Read the model definition and answer for the solid it produces. Units are mm, in the model's axes. Face numbers are marked on the shaded views. Coordinates: 2 decimals unless noted, no trailing zeros. Order: outer loops, then holes, each group sorted by start corner. A loop starts at its lowest first (then second) coordinate and runs counter-clockwise, first axis right, second up. Notation, with made-up numbers: (-13, 63.5) - (32, 63.5) arc R21 ccw to (32, 93.5) - close; hole circle Ø11 at (66, -16). An arc over 180 degrees is marked (long way). Write item = value, one per line.
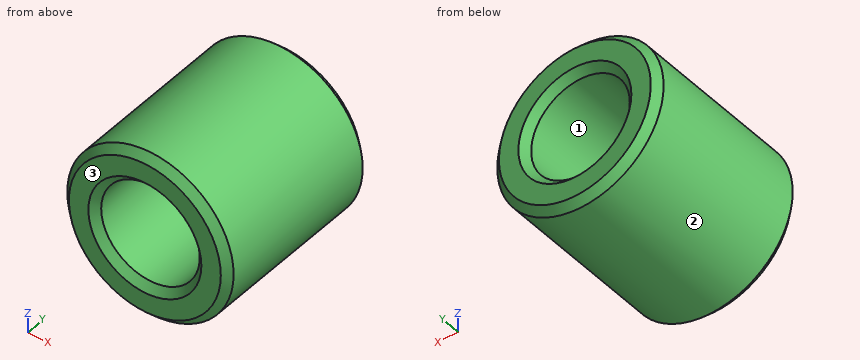
from build123d import *

# Parameters (mm, degrees)
F0_R     = 58.497005
F1_DEPTH = 127
F2_R     = 34.670049
F3_DEPTH = 127.001
F4_SIZE  = 5.08


with BuildPart() as f1:
    # F0 (on Front) → F1 (new body)
    with BuildSketch(Plane.XZ):
        Circle(F0_R)
    extrude(amount=F1_DEPTH)

    # F2 (on face) → F3 (cut, through all)
    with BuildSketch(Plane(origin=(0, 0, 0), x_dir=(-1, 0, 0), z_dir=(0, 1, 0))):
        Circle(F2_R)
    extrude(amount=-F3_DEPTH, mode=Mode.SUBTRACT)

    # F4
    f4_edges = [f1.edges().sort_by_distance(p)[0] for p in [
        (-58.497005, 0, 0),
        (34.670049, 0, 0),
        (-58.497005, -127, 0),
        (34.670049, -127, 0),
    ]]
    chamfer(f4_edges, length=F4_SIZE)


solid = f1.part
1) Determine the mould class of the marked faces 1, 2 and 3 for opening direction X: pulls with the +X half, pulls with the -X half, needs draft (parallel to the pull), parting line crosses it, or undercut.
Returned:
face_1 = undercut
face_2 = parting line crosses it
face_3 = needs draft
2) Flat-ended cylindrical pins translate along their axes: pin 1 Ø12 at (y, z) = (-82.5, -42.5) entering from +X; pin 2 Ø5 at (y, z) = (-63.5, -23.5) entering from -X; pin 3 Ø1 at (y, z) = (-95.5, 21.5) entering from +X. Find the tip coordinate at first contact, or state that the pin passes through.
Returned:
pin_1 = 45.71
pin_2 = -54.6
pin_3 = 54.6
3) The part is cut by section B-B (z = 0). Determine the outline of the cut face in (x, y), and give its area (3 significant figures).
Returned:
outline = (-58.5, -121.92) - (-53.42, -127) - (-39.75, -127) - (-34.67, -121.92) - (-34.67, -5.08) - (-39.75, 0) - (-53.42, 0) - (-58.5, -5.08) - close; (34.67, -121.92) - (39.75, -127) - (53.42, -127) - (58.5, -121.92) - (58.5, -5.08) - (53.42, 0) - (39.75, 0) - (34.67, -5.08) - close
area = 5,950 mm^2
4) The part is cut by section C-C (y = -118.5). Determine the outline of the cut face in (x, z).
Returned:
outline = circle Ø116.99 at (0, 0); hole circle Ø69.34 at (0, 0)
5) The part is cut by section A-A (x = 0). Determine the outline of the cut face in (y, z).
Returned:
outline = (-127, -53.42) - (-121.92, -58.5) - (-5.08, -58.5) - (0, -53.42) - (0, -39.75) - (-5.08, -34.67) - (-121.92, -34.67) - (-127, -39.75) - close; (-127, 39.75) - (-121.92, 34.67) - (-5.08, 34.67) - (0, 39.75) - (0, 53.42) - (-5.08, 58.5) - (-121.92, 58.5) - (-127, 53.42) - close
6) Straight lines are drawn through the part: line 1 along Z through (x, y) = (0, -35); line 2 along Z through (x, y) = (27.5, -18.5); line 3 along X through (y, z) = (-5.5, -6.5). For each, find the intervals that lie inside material, in ascending order. Write a range as from..to.
Returned:
line_1 = -58.5..-34.67, 34.67..58.5
line_2 = -51.63..-21.11, 21.11..51.63
line_3 = -58.13..-34.06, 34.06..58.13
